from build123d import *

# Parameters (mm, degrees)
SKETCH2_R      = 19.5
SKETCH2_R_2    = 4.5
SKETCH2_R_3    = 6.5
LIDBASE_DEPTH  = 2
SKETCH2_4_R    = 19.5
SKETCH2_4_R_2  = 18.5
LIDWALLS_DEPTH = 6
SKETCH3_W      = 0.5
SKETCH3_H      = 3


with BuildPart() as part:
    # Sketch2 → LidBase (new body)
    with BuildSketch(Plane(origin=(0, 0, 0), x_dir=(1, 0, 0), z_dir=(0, 1, 0))):
        Circle(SKETCH2_R)
        with Locations((0, -12)):
            Circle(SKETCH2_R_2, mode=Mode.SUBTRACT)
        Circle(SKETCH2_R_3, mode=Mode.SUBTRACT)
    extrude(amount=LIDBASE_DEPTH)

    # Sketch2<4> → LidWalls (add)
    with BuildSketch(Plane(origin=(0, 0, 0), x_dir=(1, 0, 0), z_dir=(0, 1, 0))):
        Circle(SKETCH2_4_R)
        Circle(SKETCH2_4_R_2, mode=Mode.SUBTRACT)
    extrude(amount=LIDWALLS_DEPTH)

    # Sketch3 → Beltgrooves (revolve, cut)
    with BuildSketch(Plane(origin=(0, 0, 0), x_dir=(0, 0, -1), z_dir=(1, 0, 0))):
        with Locations((19.25, 3)):
            Rectangle(SKETCH3_W, SKETCH3_H)
    revolve(axis=Axis((0, 0, 0), (0, 1, 0)), mode=Mode.SUBTRACT)


solid = part.part
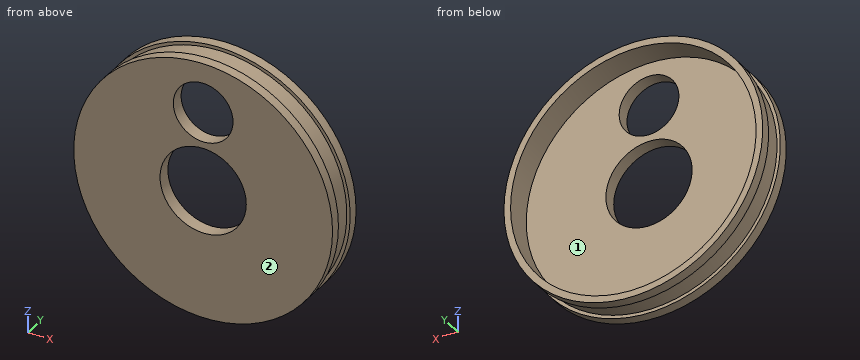
Can you work these out from the model? Positions are in its coordinate system, mm. Face numbers are marked on the shaded views. Coordinates: 2 decimals unless noted, no trailing zeros. Write each loop counter-clockwise with the first axis right and the second up, starting at its lowest first coordinate (ties: lowest second). Pieces come first, ordered by that corner, then holes. Notation, with made-up numbers: (-1, 27) - (14, 27) arc R31 cw to (14, 53) - close; hole circle Ø4 at (83, 4). An arc over 180 degrees is marked (long way). Return JSON: item names as keys, results as strings. Group by question number.
Item 1: Please list where these lines run through material, in increasing order: probe 1 along Z at (x, y) = (0, 0.75); probe 2 along X at (y, z) = (0.5, 0); probe 3 along Z at (x, y) = (0, 4.45).
Item 2: If we section it at A-A (z = 0): Write out the boundary of the cut face in (x, y), then the cut area to 3 significant figures.
Item 3: If we section it at D-D (y = 5.2): Write out the boundary of the cut face in (x, z).
Item 4: We'd pull the mould along X, two halves only. Please class the marked faces 1 and 2: pulls with the +X half, pulls with the -X half, needs draft (parallel to the pull), parting line crosses it, or undercut.
Item 5: I'm going to push flat-ended pins straight in: pin 1 Ø5.5 at (x, z) = (0, 12) entering from +Y; pin 2 Ø1 at (x, y) = (15.5, 3.5) entering from -Z; pin 3 Ø18.5 at (x, z) = (-5, 2.5) entering from +Y; pin 4 Ø3 at (x, y) = (-12.5, 5) entering from -Z. Where does each tip first touch, or does it pass through?
Item 6: If we section it at C-C (x = 13): Write out the boundary of the cut face in (y, z), then the cut area to 3 significant figures.
Item 7: If we section it at B-B (x = 0): Write out the boundary of the cut face in (y, z), then the cut area to 3 significant figures.
Return value:
{
 "1": {"probe 1": "z = -19.5 to -6.5, 6.5 to 7.5, 16.5 to 19.5", "probe 2": "x = -19.5 to -6.5, 6.5 to 19.5", "probe 3": "z = -19 to -18.5, 18.5 to 19"},
 "2": {"outline": "(-19.5, 0) - (-6.5, 0) - (-6.5, 2) - (-18.5, 2) - (-18.5, 6) - (-19.5, 6) - (-19.5, 4.5) - (-19, 4.5) - (-19, 1.5) - (-19.5, 1.5) - close; (6.5, 0) - (19.5, 0) - (19.5, 1.5) - (19, 1.5) - (19, 4.5) - (19.5, 4.5) - (19.5, 6) - (18.5, 6) - (18.5, 2) - (6.5, 2) - close", "area": "57.0 mm^2"},
 "3": {"outline": "circle Ø39 at (0, 0); hole circle Ø37 at (0, 0)"},
 "4": {"face 1": "undercut", "face 2": "needs draft"},
 "5": {"pin 1": "passes through", "pin 2": "stops at z = -11.66", "pin 3": "stops at y = 2", "pin 4": "stops at z = -16.1"},
 "6": {"outline": "(0, -14.53) - (1.5, -14.53) - (1.5, -13.86) - (4.5, -13.86) - (4.5, -14.53) - (6, -14.53) - (6, -13.16) - (2, -13.16) - (2, 13.16) - (6, 13.16) - (6, 14.53) - (4.5, 14.53) - (4.5, 13.86) - (1.5, 13.86) - (1.5, 14.53) - (0, 14.53) - close", "area": "65.0 mm^2"},
 "7": {"outline": "(0, -19.5) - (1.5, -19.5) - (1.5, -19) - (4.5, -19) - (4.5, -19.5) - (6, -19.5) - (6, -18.5) - (2, -18.5) - (2, -6.5) - (0, -6.5) - close; (0, 6.5) - (2, 6.5) - (2, 7.5) - (0, 7.5) - close; (0, 16.5) - (2, 16.5) - (2, 18.5) - (6, 18.5) - (6, 19.5) - (4.5, 19.5) - (4.5, 19) - (1.5, 19) - (1.5, 19.5) - (0, 19.5) - close", "area": "39.0 mm^2"}
}
